Drawing for the job (mm, zero at the part's lowest x, y, z). A direction names the side the tool comes from. Give positions to 0.01 mm unless a question says otherwise; leave off trailing zeros. Order: outer loops, then holes, each group sorted by start corner. A loop starts at its lowest first (then second) coordinate and runs counter-clockwise, first axis right, second up. Notation, with made-up numbers: (4, 67.25) - (30, 67.25) arc R20 cw to (30, 89.25) - close; hole circle Ø3 at (-37, 13). An arc over 180 degrees is marked (long way). One line per item, written item: value.
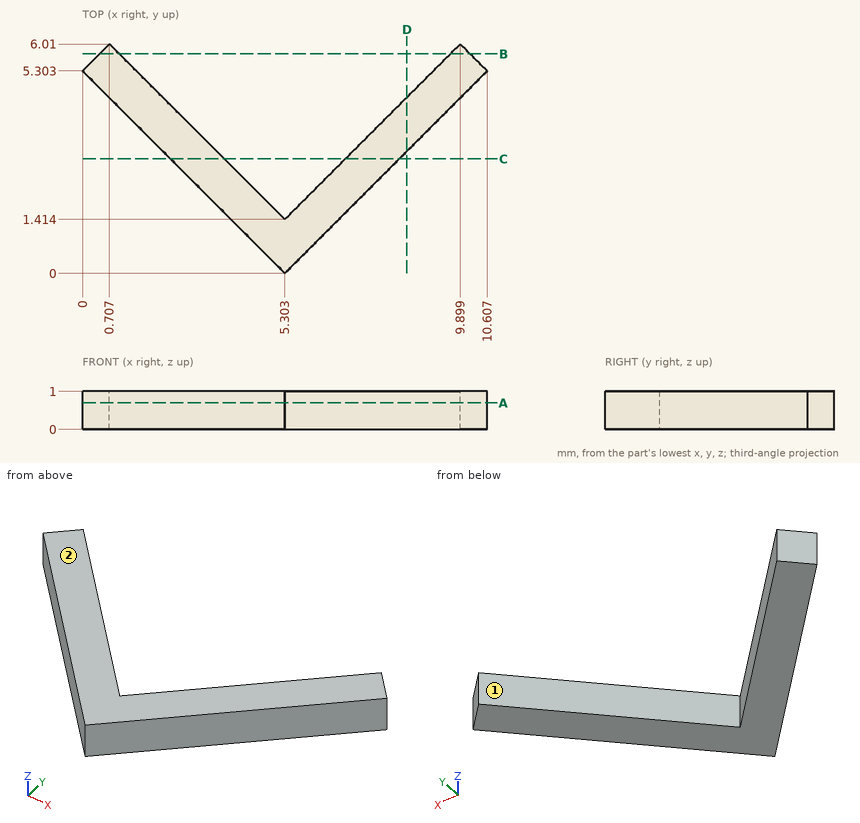
1) Cut at D-D, the plane x = 8.5. Give the cut face in (y, z).
Outcome:
outline: (3.2, 0) - (4.61, 0) - (4.61, 1) - (3.2, 1) - close
2) Cut at C-C, the plane y = 3. Give the cut face in (x, z).
Outcome:
outline: (2.3, 0) - (3.72, 0) - (3.72, 1) - (2.3, 1) - close; (6.89, 0) - (8.3, 0) - (8.3, 1) - (6.89, 1) - close
3) Drill centre lines: line 1 along X through (y, z) = (1.5, 0.9) (1 decimal); line 2 along X through (y, z) = (3, 0.45) (1 decimal); line 3 along X through (y, z) = (1.25, 0.85) (1 decimal). Where is each one in solid material? Low to high. Write a range as from..to.
Outcome:
line 1: x = 3.8..5.2, 5.4..6.8
line 2: x = 2.3..3.7, 6.9..8.3
line 3: x = 4.1..6.6
4) Cut at B-B, the plane y = 5.75. Give the cut face in (x, z).
Outcome:
outline: (0.45, 0) - (0.97, 0) - (0.97, 1) - (0.45, 1) - close; (9.64, 0) - (10.16, 0) - (10.16, 1) - (9.64, 1) - close
5) Cut at A-A, the plane z = 0.7. Give the cut face in (x, y) (1 decimal), then the cut area to 3 significant figures.
Outcome:
outline: (0, 5.3) - (5.3, 0) - (10.6, 5.3) - (9.9, 6) - (5.3, 1.4) - (0.7, 6) - close
area: 14.0 mm^2
6) Which spindle directions (+Z, -Z, +X, -X, +Y, -Y) get a long thin tool onto all of the face, cutting with end or side? Do the marked faces 1 and 2. Say none if no direction does.
Outcome:
face 1: +Z, -Z, +Y
face 2: +Z, +X, -X, +Y, -Y
